Read the model definition and answer for the solid it produces. Units are mm, in the model's axes. Coordinates: 2 decimals unless noted, no trailing zeros. Write each loop counter-clockwise with the first axis right and the second up, starting at its lowest first coordinate (ties: lowest second). Pieces come first, ordered by that corner, then holes.
(1) Section D-D on x = 1.65 is taken. Write down the section's boundary in (y, z), then the cut area to 3 significant figures.
(2) Find the intervals of material crossed by probe 1 along Y at (x, z) = (1.25, 3.25); probe 2 along Y at (x, z) = (2.2, 7.5); probe 3 along X at (y, z) = (0.55, 7.5), in increasing order.
(3) Section A-A on x = 1.25 is taken. Write down the section's boundary in (y, z).
(4) Section C-C on x = 0.8 is taken. Write down the section's boundary in (y, z), then the cut area to 3 significant figures.
(5) Section B-B on z = 1.25 is taken. Write down the section's boundary in (x, y), then the cut area to 3 significant figures.
from build123d import *

# Parameters (mm, degrees)
SKETCH_R  = 0.25
PAD_DEPTH = 10


with BuildPart() as part:
    # Sketch → Pad (new body)
    with BuildSketch(Plane.XY):
        with BuildLine():
            Line((0, 0), (0, -2.1))
            Line((0, -2.1), (2.5, -2.1))
            Line((2.5, -2.1), (2.5, 0))
            ThreePointArc((2.5, 0), (1.25, 1.25), (0, 0))
        make_face()
        with Locations((1.25, 0)):
            Circle(SKETCH_R, mode=Mode.SUBTRACT)
    extrude(amount=PAD_DEPTH)


solid = part.part
Response:
1. outline: (-2.1, 0) - (1.18, 0) - (1.18, 10) - (-2.1, 10) - close
1. area: 32.8 mm2
2. probe 1: y = -2.1 to -0.25, 0.25 to 1.25
2. probe 2: y = -2.1 to 0.81
2. probe 3: x = 0.13 to 2.37
3. outline: (-2.1, 0) - (-0.25, 0) - (-0.25, 10) - (-2.1, 10) - close; (0.25, 0) - (1.25, 0) - (1.25, 10) - (0.25, 10) - close
4. outline: (-2.1, 0) - (1.17, 0) - (1.17, 10) - (-2.1, 10) - close
4. area: 32.7 mm2
5. outline: (0, -2.1) - (2.5, -2.1) - (2.5, 0) arc R1.25 ccw to (0, 0) - close; hole circle Ø0.5 at (1.25, 0)
5. area: 7.51 mm2
